Source: CAD feature listing. Evaluate the final solid. Frame: model axes, mm. A direction names the side the tool comes from. Give positions to 0.01 mm unless a question says otherwise; leave off trailing zeros. Loops run counter-clockwise (first coordinate to the right, second up) from the corner with the lowest first, then second, coordinate; pieces in that order, holes last.
```python
from build123d import *

# Parameters (mm, degrees)
BOSS_EXTRUDE1_DEPTH = 25
SKETCH5_W           = 14.15
SKETCH5_H           = 14.15
CUT_EXTRUDE4_DEPTH  = 346.591241967
CUT_EXTRUDE5_REACH  = 371.537
SKETCH6_R           = 1.775
BOSS_EXTRUDE2_DEPTH = 25
SKETCH9_R           = 1.775
CUT_EXTRUDE6_DEPTH  = 15.926403812


with BuildPart() as part:
    # Sketch1 → Boss-Extrude1 (new body)
    with BuildSketch(Plane(origin=(0, 0, 0), x_dir=(0, 0, -1), z_dir=(1, 0, 0))):
        Polygon((-75.827871616, -173.427267807), (-55.827871616, -173.427267807), (-55.827871616, -191.427267807), (-130.827871616, -336.427267807), (-150.827871616, -336.427267807), (-91.827871616, -222.360601141), (-75.827871616, -191.427267807), align=None)
    extrude(amount=BOSS_EXTRUDE1_DEPTH)

    # Sketch5 → Cut-Extrude4 (cut, through all)
    with BuildSketch(Plane.XY.offset(75.827871616)):
        with Locations((12.5, -180.502267807)):
            Rectangle(SKETCH5_W, SKETCH5_H)
    extrude(amount=-CUT_EXTRUDE4_DEPTH, mode=Mode.SUBTRACT)

    # Cut-Extrude5: up to this face of the body (flat: up to its plane)
    cut_extrude5_end = Plane(part.part.faces().sort_by_distance((0, -254.927267807, 99.186767321))[0])
    # Sketch6 → Cut-Extrude5 (cut, up to the picked face)
    with BuildSketch(Plane(origin=(25, 0, 0), x_dir=(0, 0, -1), z_dir=(1, 0, 0)), mode=Mode.PRIVATE) as cut_extrude5_sk1:
        with Locations((-68.827871616, -180.477267807)):
            Circle(SKETCH6_R)
    cut_extrude5_tool1 = split(extrude(cut_extrude5_sk1.sketch, amount=-CUT_EXTRUDE5_REACH, mode=Mode.PRIVATE), bisect_by=cut_extrude5_end, keep=Keep.BOTH, mode=Mode.PRIVATE)
    add(cut_extrude5_tool1.solids().sort_by(Axis((25, -180.477268, 68.827872), (-1, 0, 0)))[0], mode=Mode.SUBTRACT)

    # Sketch8 → Boss-Extrude2 (add)
    with BuildSketch(Plane(origin=(25, 0, 0), x_dir=(0, 0, -1), z_dir=(1, 0, 0))):
        Polygon((-126.827871616, -187.577267807), (-116.827871616, -187.577267807), (-116.827871616, -196.577267807), (-107.00799507, -196.577267807), (-89.793388857, -218.427267807), (-95.84798887, -230.132827833), (-116.827871616, -203.503671619), (-126.827871616, -203.503671619), (-126.827871616, -196.577267807), align=None)
    extrude(amount=-BOSS_EXTRUDE2_DEPTH)

    # Sketch9 → Cut-Extrude6 (cut)
    with BuildSketch(Plane(origin=(0, -187.577267807, 0), x_dir=(1, 0, 0), z_dir=(0, 1, 0))):
        with Locations(Location((12.5, -121.827871616, 0), (0, 0, 270))):
            Circle(SKETCH9_R)
    extrude(amount=-CUT_EXTRUDE6_DEPTH, mode=Mode.SUBTRACT)


solid = part.part
```
(1) Section D-D, the plane y = -277.5. Return the cut outline in (x, z), then the cut area to 3 significant figures.
A:
outline: (0, 100.35) - (25, 100.35) - (25, 120.35) - (0, 120.35) - close
area: 500 mm2
(2) Section B-B, the plane y = -215. Return the cut outline in (x, z), then the cut area to 3 significant figures.
A:
outline: (0, 68.02) - (25, 68.02) - (25, 88.02) - (0, 88.02) - close; (0, 92.49) - (25, 92.49) - (25, 107.77) - (0, 107.77) - close
area: 882 mm2
(3) Ray query, line 1 along Z through (x, y) = (13.75, -189); line 2 along Z through (x, y) = (21, -188); line 3 along Y through (x, z) = (5, 119). Return the intervals inside material, ascending.
A:
line 1: z = 55.83 to 75.83, 116.83 to 120.57, 123.09 to 126.83
line 2: z = 55.83 to 75.83, 116.83 to 126.83
line 3: y = -313.56 to -274.89, -203.5 to -187.58
(4) Mould query, pull axis Y, two halves, no side actions, for faces 1 (the flat face through (12, -336.427, 141)), 2 (the cylindrical face through (2.75, -178.981, 67.874)), 3 (the flat face through (5.425, -181, 66)), 4 (the flat face through (12, -187.577, 66)). Classes: pulls with the +Y half, pulls with the -Y half, needs draft (parallel to the pull), parting line crosses it, or undercut.
A:
face 1: pulls with the -Y half
face 2: undercut
face 3: needs draft
face 4: pulls with the +Y half
(5) Reachability of faces 5 (the flat face through (12.7, -187.577, 119.7)), 6 (the flat face through (12.7, -203.504, 119.5)), 7 (the flat face through (19.575, -181, 66)) from +Z, -Z, +X, -X, +Y, -Y: full face, straight path, thin tool, end or side. Return the list, or none.
A:
face 5: +Z, +X, -X, +Y
face 6: +Z, +X, -X
face 7: +Z, -Z, +Y
(6) Section A-A, the plane x = 12.5. Return the cut outline in (y, z), then the cut area to 3 significant figures.
A:
outline: (-336.43, 130.83) - (-191.43, 55.83) - (-187.58, 55.83) - (-187.58, 75.83) - (-191.43, 75.83) - (-218.43, 89.79) - (-196.58, 107.01) - (-196.58, 116.83) - (-187.58, 116.83) - (-187.58, 120.05) - (-203.5, 120.05) - (-203.5, 116.83) - (-230.13, 95.85) - (-336.43, 150.83) - close; (-203.5, 123.6) - (-187.58, 123.6) - (-187.58, 126.83) - (-203.5, 126.83) - close
area: 3,480 mm2
(7) First-contact query: pin 1 (6 mm diameter, centred on x = 6, z = 91.5, fed in from +Y); pin 2 (2 mm diameter, centred on y = -180.48, z = 68.83, fed in from -X); pin 3 (11 mm diameter, centred on x = 8, z = 123.5, fed in from +Y); pin 4 (5 mm diameter, centred on x = 15.5, z = 122, fed in from -Y). Flat tips, straight axial feed; report the tip coordinate or a pass-through.
A:
pin 1: stops at y = -212.45
pin 2: passes through
pin 3: stops at y = -187.58
pin 4: stops at y = -324.19
(8) Section C-C, the plane x = 21.5. Return the cut outline in (y, z) (3 decimals).
A:
outline: (-336.427, 130.828) - (-191.427, 55.828) - (-173.427, 55.828) - (-173.427, 75.828) - (-191.427, 75.828) - (-218.427, 89.793) - (-196.577, 107.008) - (-196.577, 116.828) - (-187.577, 116.828) - (-187.577, 126.828) - (-203.504, 126.828) - (-203.504, 116.828) - (-230.133, 95.848) - (-336.427, 150.828) - close; hole circle Ø3.55 at (-180.477, 68.828)
